from build123d import *

# Parameters (mm, degrees)
BOSS_EXTRUDE1_DEPTH = 2.5
SKETCH2_R           = 5
BOSS_EXTRUDE2_DEPTH = 1
FILLET1_R           = 1
M5_TAPPED_HOLE1_D   = 4.2
M4_TAPPED_HOLE1_D   = 3.3


with BuildPart() as part:
    # Sketch1 → Boss-Extrude1 (new, symmetric)
    with BuildSketch(Plane.XY):
        with BuildLine():
            Line((-5.5, 19.228884523), (-20, 0))
            ThreePointArc((-20, 0), (0, -20), (20, 0))
            Line((20, 0), (5.5, 19.228884523))
            ThreePointArc((5.5, 19.228884523), (0, 20), (-5.5, 19.228884523))
        make_face()
    extrude(amount=BOSS_EXTRUDE1_DEPTH, both=True)

    # Sketch2 → Boss-Extrude2 (add)
    with BuildSketch(Plane(origin=(0, 0, -2.5), x_dir=(-1, 0, 0), z_dir=(0, 0, -1))):
        Circle(SKETCH2_R)
    extrude(amount=BOSS_EXTRUDE2_DEPTH)

    # Fillet1
    fillet1_edges = [part.edges().sort_by_distance(p)[0] for p in [
        (5, 0, -2.5),
    ]]
    fillet(fillet1_edges, radius=FILLET1_R - 0.0001)  # a hair under: the kernel refuses the full size

    # M5 Tapped Hole1 (through all)
    with Locations(Plane.XY.offset(2.5)):
        with Locations((0, 0)):
            Hole(M5_TAPPED_HOLE1_D / 2)

    # M4 Tapped Hole1 (through all)
    with Locations(Plane(origin=(0, 13, 2.5), x_dir=(1, 0, 0), z_dir=(0, 0, 1))):
        with Locations((0, 0)):
            Hole(M4_TAPPED_HOLE1_D / 2)


solid = part.part
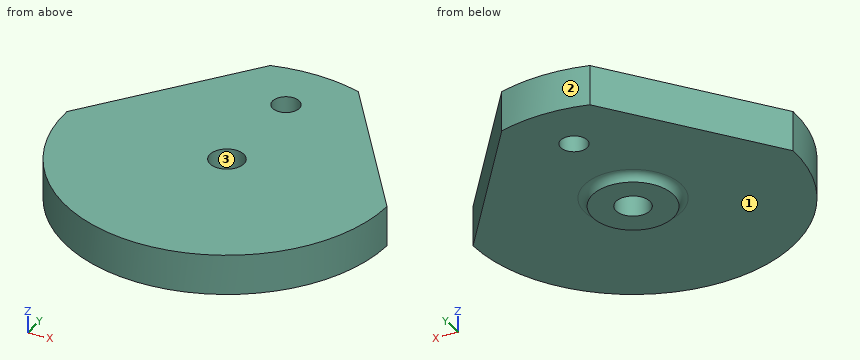
Geometry check sheet. Reference: the model listing, model coordinates, mm. Face numbers are marked on the shaded views. Give positions to 0.01 mm unless a question says otherwise; leave off trailing zeros. Order: outer loops, then holes, each group sorted by start corner. A loop starts at its lowest first (then second) coordinate and runs counter-clockwise, first axis right, second up. Notation, with made-up numbers: (76, 24.25) - (87, 24.25) arc R29 ccw to (87, 50.25) - close; hole circle Ø2 at (87.25, -39.5). An arc over 180 degrees is marked (long way). Use one line per item in the form item = value.
1) Depth check by flat-ended pin: pin 1 Ø2.5 at (x, y) = (0, 13) entering from -Z (3 decimals); pin 2 Ø3 at (y, z) = (15, -1) entering from -X; pin 3 Ø1.5 at (x, z) = (-7, 1.5) entering from -Y; pin 4 Ø1.5 at (y, z) = (-0.5, -2) entering from +X. Enter the tip coordinate at first touch or a pass-through.
Working result:
pin_1 = through
pin_2 = -9.82
pin_3 = -19
pin_4 = 20
2) Sectioned sample at D-D (x = 8.5). Record the boundary of the cut face in (y, z).
Working result:
outline = (-18.1, -2.5) - (15.25, -2.5) - (15.25, 2.5) - (-18.1, 2.5) - close
3) Draft check along X on the marked faces 1, 2 and 3. Enter one of: released by +X, released by -X, zero draft, split by the parting line, or undercut.
Working result:
face_1 = zero draft
face_2 = split by the parting line
face_3 = undercut
4) Material ranges on probe 1 along Y at (x, z) = (0, 1.45); probe 2 along Z at (x, y) = (-16, -10); probe 3 along X at (y, z) = (14, 0.3), recorded low to high. Write a range as from..to.
Working result:
probe_1 = -20..-2.1, 2.1..11.35, 14.65..20
probe_2 = -2.5..2.5
probe_3 = -9.44..-1.31, 1.31..9.44
5) Sectioned sample at A-A (x = 0). Count the separate pieces of the cut face and the enclosed holes in it, and give its area (3 significant figures).
Working result:
separate_pieces = 3
enclosed_holes = 0
area = 169 mm^2
6) Sectioned sample at C-C (z = -0.7). Record the boundary of the cut face in (x, y), and give its area (3 significant figures).
Working result:
outline = (-20, 0) arc R20 ccw to (20, 0) - (5.5, 19.23) arc R20 ccw to (-5.5, 19.23) - close; hole circle Ø4.2 at (0, 0); hole circle Ø3.3 at (0, 13)
area = 1,100 mm^2
7) Sectioned sample at B-B (y = 13). Record the boundary of the cut face in (x, z), and give its area (3 significant figures).
Working result:
outline = (-10.2, -2.5) - (-1.65, -2.5) - (-1.65, 2.5) - (-10.2, 2.5) - close; (1.65, -2.5) - (10.2, -2.5) - (10.2, 2.5) - (1.65, 2.5) - close
area = 85.5 mm^2
